Here's how the part is built. I have some questions about the finished solid (model axes, mm). A direction names the side the tool comes from. Give positions to 0.01 mm unless a question says otherwise; leave off trailing zeros. Write each loop counter-clockwise with the first axis right and the second up, starting at its lowest first coordinate (ties: lowest second). Pieces come first, ordered by that corner, then holes. Notation, with made-up numbers: M 45.5,56 L 89.5,56 A33 cw 89.5,91 Z; hole C 76,24.5 d2. An arc over 180 degrees is marked long. Answer as CSV lines item,"result". Start each with the question number.
Q1. For pin 1 (1 mm diameter, centred on x = 10.5, y = 6, fed in from -Z); pin 2 (10 mm diameter, centred on y = -6, z = 20.5, fed in from -X); pin 3 (1.6 mm diameter, centred on x = 0, y = 0.5, fed in from +Z), each with a flat end and sliding along its axis, tell me the tip position at first contact or that it passes through.
Q2. Suppose I cut it at A-A (y = 11.5). Write out the boundary of the cut face in (x, z).
Q3. Suppose I cut it at D-D (z = -15). Write out the boundary of the cut face in (x, y).
Q4. Thinking about a two-plate mould opening in X: for faces 1 (the cylindrical face through (-1.27, 0.97, -29.45)), 2 (the cylindrical face through (-11.74, 0.39, 20.96)), 3 (the flat face through (-1.3, 1.3, 26.388)), which applies, +X half, -X half, draft (parallel to the pull), parting line (faces both ways), or undercut?
Q5. On a 3-axis mill with a long thin cutter (end or side, diameter ignored), from which of +Z, -Z, +X, -X, +Y, -Y can I reach the whole of each face in a straight line? I mean faces 4 (the flat face through (0, 2, 33.588)), 5 (the flat face through (3, 3, 27.388)), 6 (the flat face through (-2, 0, -26)), 7 (the flat face through (2, 0, 26)). Say none if no direction works.
Q6. Suppose I cut it at B-B (x = -8). Write out the boundary of the cut face in (y, z).
Q7. Suppose I cut it at C-C (z = -27). Write out the boundary of the cut face in (x, y).
Q8. If I drill on line 1 along X through (y, z) = (0, 21); line 2 along Z through (x, y) = (-2, -1); line 3 along Z through (x, y) = (5, 2), over which ranges is the centre line in solid material (lowest first)?
```python
from build123d import *

# Parameters (mm, degrees)
F3_D     = 2.6
F3_DEPTH = 5
F3_TIP   = 0.7811188047


with BuildPart() as f1:
    # F0 (on Front) → F1 (revolve)
    with BuildSketch(Plane.XZ):
        Polygon((1.6, 33), (0, 33), (0, -33), (1.6, -33), (1.6, -26), (4.925, -26), (4.925, -23.5), (15.25, -23.5), (15.25, -6.5), (16.25, -6.5), (16.25, 18.5), (15.25, 18.5), (15.25, 23.5), (4.925, 23.5), (4.925, 26), (1.6, 26), align=None)
    revolve(axis=Axis((0, 0, 0), (0, 0, -1)))

    # F3
    with Locations(Plane.XY.offset(23.5)):
        with Locations((-10.5, 0), (10.5, 0)):
            Hole(F3_D / 2, depth=F3_DEPTH)
            with Locations((0, 0, -(F3_DEPTH + F3_TIP / 2))):  # 118° drill point
                Cone(0, F3_D / 2, F3_TIP, mode=Mode.SUBTRACT)

    # F4 (on Front) → F5 (revolve)
    with BuildSketch(Plane.XZ):
        Polygon((3.875, 27.3875447527), (3.875, 33.5875447527), (1.6, 33.5875447527), (1.6, 26.3875447527), (6.4063321701, 26.3875447527), (6.4063321701, 27.3875447527), align=None)
    revolve(axis=Axis((0, 0, 0), (0, 0, -1)))


solid = f1.part
```
Resolved:
1,pin 1,"z = -23.5"
1,pin 2,"x = -16.19"
1,pin 3,"z = 33"
2,outline,"M -11.48,-6.5 L -10.02,-6.5 L -10.02,-23.5 L 10.02,-23.5 L 10.02,-6.5 L 11.48,-6.5 L 11.48,18.5 L 10.02,18.5 L 10.02,23.5 L -10.02,23.5 L -10.02,18.5 L -11.48,18.5 Z"
3,outline,"C 0,0 d30.5"
4,face 1,"parting line"
4,face 2,"undercut"
4,face 3,"draft"
5,face 4,"+Z, +X, -X, +Y, -Y"
5,face 5,"+Z"
5,face 6,"-Z"
5,face 7,"none"
6,outline,"M -14.14,-6.5 L -12.98,-6.5 L -12.98,-23.5 L 12.98,-23.5 L 12.98,-6.5 L 14.14,-6.5 L 14.14,18.5 L 12.98,18.5 L 12.98,23.5 L -12.98,23.5 L -12.98,18.5 L -14.14,18.5 Z"
7,outline,"C 0,0 d3.2"
8,line 1,"-15.25 to -11.8, -9.2 to 9.2, 11.8 to 15.25"
8,line 2,"-26 to 26, 26.39 to 33.59"
8,line 3,"-23.5 to 23.5, 26.39 to 27.39"
